Can you work these out from the model? Positions are in its coordinate system, mm. Face numbers are marked on the shaded views. A direction names the side the tool comes from. Round coordinates to 2 decimals unless told otherwise and drop trailing zeros. Loops run counter-clockwise (first coordinate to the right, second up) from the corner with the lowest first, then second, coordinate; pieces in that order, holes last. Notation, with made-up numbers: (33.5, 2.25) -> (89.5, 2.25) arc R21 cw to (89.5, 8.25) -> close; hole circle Ø6 at (14, 46.25). An arc over 180 degrees is marked (long way). Use a Markdown table: item, result.
from build123d import *

# Parameters (mm, degrees)
SKETCH_3_W           = 180
SKETCH_3_H           = 43
EXTRUDE_1_DEPTH      = 12
CUT_EXTRUDE_1_DEPTH  = 52
CUT_EXTRUDE_2_DEPTH  = 5
CUT_EXTRUDE_3_DEPTH  = 5
SKETCH_8_W           = 55
SKETCH_8_H           = 37
CUT_EXTRUDE_4_DEPTH  = 10.5
CUT_EXTRUDE_5_DEPTH  = 3
SKETCH_10_W          = 62.128790526
SKETCH_10_H          = 8.683746703
CUT_EXTRUDE_6_DEPTH  = 8
CUT_EXTRUDE_8_DEPTH  = 9
FILLET_2_R           = 2
FILLET_3_R           = 3
SKETCH_12_W          = 20
SKETCH_12_H          = 16
EXTRUDE_2_DEPTH      = 2
SKETCH_13_W          = 16
SKETCH_13_H          = 5
CUT_EXTRUDE_9_DEPTH  = 1
SKETCH_14_W          = 10
SKETCH_14_H          = 4.5
CUT_EXTRUDE_10_DEPTH = 11
EXTRUDE_3_DEPTH      = 2
EXTRUDE_3_DEPTH_BACK = 3
SKETCH_15_W          = 4.878003414
SKETCH_15_H          = 8.248491994


with BuildPart() as part:
    # 草图3 → 凸台-拉伸1 (new body)
    with BuildSketch(Plane(origin=(0, 0, 0), x_dir=(1, 0, 0), z_dir=(0, 1, 0))):
        with Locations((50.068597249, 7.753123643)):
            Rectangle(SKETCH_3_W, SKETCH_3_H)
    extrude(amount=EXTRUDE_1_DEPTH)

    # 草图4 → 切除-拉伸1 (cut)
    with BuildSketch(Plane(origin=(0, 0, 0), x_dir=(1, 0, 0), z_dir=(0, 1, 0))):
        Polygon((-22.469613434, -5.858946979), (26.002261286, -5.858946979), (29.068597249, -13.746876357), (-25.931402751, -13.746876357), align=None)
    extrude(amount=CUT_EXTRUDE_1_DEPTH, mode=Mode.SUBTRACT)

    # 草图5 → 切除-拉伸2 (cut)
    with BuildSketch(Plane(origin=(0, 12, 0), x_dir=(1, 0, 0), z_dir=(0, 1, 0))):
        Polygon((140.068597249, 7.753123643), (140.068597249, 22.753123643), (125.276479966, 22.753123643), (125.276479966, -7.246876357), (140.068597249, -7.246876357), align=None)
    extrude(amount=-CUT_EXTRUDE_2_DEPTH, mode=Mode.SUBTRACT)

    # 草图7 → 切除-拉伸3 (cut)
    with BuildSketch(Plane(origin=(0, 12, 0), x_dir=(1, 0, 0), z_dir=(0, 1, 0))):
        Polygon((125.276479966, 7.753123643), (125.276479966, 25.753123643), (100.500825538, 25.753123643), (100.500825538, -10.246876357), (125.276479966, -10.246876357), align=None)
    extrude(amount=-CUT_EXTRUDE_3_DEPTH, mode=Mode.SUBTRACT)

    # 草图8 → 切除-拉伸4 (cut)
    with BuildSketch(Plane(origin=(0, 12, 0), x_dir=(1, 0, 0), z_dir=(0, 1, 0))):
        with Locations((63.776287419, 7.753123643)):
            Rectangle(SKETCH_8_W, SKETCH_8_H)
    extrude(amount=-CUT_EXTRUDE_4_DEPTH, mode=Mode.SUBTRACT)

    # 草图9 → 切除-拉伸5 (cut)
    with BuildSketch(Plane(origin=(0, 12, 0), x_dir=(1, 0, 0), z_dir=(0, 1, 0))):
        Polygon((91.276287419, 26.253123643), (96.635770173, 26.253123643), (96.635770173, 22.130591531), (96.635770173, 13.862098754), (97.813575381, 11.877191358), (100.500825538, 11.877191358), (100.500825538, 3.393971617), (96.236747254, 3.393971617), (92.132656028, 10.310430274), (92.132656028, 21.255120764), (91.276287419, 21.255120764), align=None)
    extrude(amount=-CUT_EXTRUDE_5_DEPTH, mode=Mode.SUBTRACT)

    # 草图10 → 切除-拉伸6 (cut)
    with BuildSketch(Plane(origin=(0, 12, 0), x_dir=(1, 0, 0), z_dir=(0, 1, 0))):
        with Locations((1.934159822, -6.405003006)):
            Rectangle(SKETCH_10_W, SKETCH_10_H)
    extrude(amount=-CUT_EXTRUDE_6_DEPTH, mode=Mode.SUBTRACT)

    # 草图11 → 切除-拉伸8 (cut)
    with BuildSketch(Plane(origin=(0, 12, 0), x_dir=(1, 0, 0), z_dir=(0, 1, 0))):
        Polygon((32.998555085, -10.746876357), (-36.5396752, -10.746876357), (-36.5396752, 26.253123643), (36.276287419, 26.253123643), (36.276287419, -2.167243749), (32.998555085, -2.063129654), align=None)
    extrude(amount=-CUT_EXTRUDE_8_DEPTH, mode=Mode.SUBTRACT)

    # 圆角2
    fillet_2_edges = [part.edges().sort_by_distance(p)[0] for p in [
        (84.568597249, 0, 13.746876357),
        (-24.200508092, 0, 9.802911668),
        (27.535429268, 0, 9.802911668),
        (50.068597249, 0, -29.253123643),
        (140.068597249, 0, -7.753123643),
        (-32.931402751, 0, 13.746876357),
        (-39.931402751, 0, -7.753123643),
    ]]
    fillet(fillet_2_edges, radius=FILLET_2_R)

    # 圆角3
    # the kernel refuses this fillet: 3 mm, written as the material it takes off along each edge
    with BuildSketch(Plane(origin=(-36.931402751, 0, 10.746876357), x_dir=(0, 0, 1), z_dir=(1, 0, 0))) as fillet_3_piece_1:
        with BuildLine():
            CenterArc((1, -2), 2, 0, 90)
            Line((3, -2), (3, 0))
            Line((3, 0), (1, 0))
        make_face()
    revolve(axis=Axis((-36.931402751, 0, 10.746876357), (0, -1, 0)), revolution_arc=90, mode=Mode.SUBTRACT)
    with BuildSketch(Plane(origin=(-36.931402751, 0, -26.253123643), x_dir=(-1, 0, 0), z_dir=(0, 0, 1))) as fillet_3_piece_2:
        with BuildLine():
            CenterArc((1, -2), 2, 0, 90)
            Line((3, -2), (3, 0))
            Line((3, 0), (1, 0))
        make_face()
    revolve(axis=Axis((-36.931402751, 0, -26.253123643), (0, -1, 0)), revolution_arc=90, mode=Mode.SUBTRACT)
    with BuildSketch(Plane(origin=(137.068597249, 0, 10.746876357), x_dir=(1, 0, 0), z_dir=(0, 0, -1))) as fillet_3_piece_3:
        with BuildLine():
            CenterArc((1, -2), 2, 0, 90)
            Line((3, -2), (3, 0))
            Line((3, 0), (1, 0))
        make_face()
    revolve(axis=Axis((137.068597249, 0, 10.746876357), (0, -1, 0)), revolution_arc=90, mode=Mode.SUBTRACT)
    with BuildSketch(Plane(origin=(137.068597249, 0, -26.253123643), x_dir=(0, 0, -1), z_dir=(-1, 0, 0))) as fillet_3_piece_4:
        with BuildLine():
            CenterArc((1, -2), 2, 0, 90)
            Line((3, -2), (3, 0))
            Line((3, 0), (1, 0))
        make_face()
    revolve(axis=Axis((137.068597249, 0, -26.253123643), (0, -1, 0)), revolution_arc=90, mode=Mode.SUBTRACT)
    with BuildSketch(Plane(origin=(-39.931402751, 0, -29.253123643), x_dir=(1, 0, 0), z_dir=(0, 1, 0))) as fillet_3_piece_5:
        with BuildLine():
            CenterArc((FILLET_3_R, -FILLET_3_R), FILLET_3_R, 90, 90)
            Line((0, -FILLET_3_R), (0, 0))
            Line((0, 0), (FILLET_3_R, 0))
        make_face()
    extrude(amount=19.5, mode=Mode.SUBTRACT)
    with BuildSketch(Plane(origin=(140.068597249, 0, -29.253123643), x_dir=(-1, 0, 0), z_dir=(0, 1, 0)), Plane(origin=(140.068597249, 0, 13.746876357), x_dir=(0, 0, -1), z_dir=(0, 1, 0)), Plane(origin=(-39.931402751, 0, 13.746876357), x_dir=(1, 0, 0), z_dir=(0, 1, 0))) as fillet_3_piece_6:
        with BuildLine():
            CenterArc((FILLET_3_R, FILLET_3_R), FILLET_3_R, 180, 90)
            Line((0, FILLET_3_R), (0, 0))
            Line((0, 0), (FILLET_3_R, 0))
        make_face()
    extrude(amount=19.5, mode=Mode.SUBTRACT)

    # 草图12 → 凸台-拉伸2 (add)
    with BuildSketch(Plane(origin=(0, 3, 0), x_dir=(1, 0, 0), z_dir=(0, 1, 0))):
        with Locations((-26.5396752, 11.082072108)):
            Rectangle(SKETCH_12_W, SKETCH_12_H)
    extrude(amount=EXTRUDE_2_DEPTH)

    # 草图13 → 切除-拉伸9 (cut)
    with BuildSketch(Plane(origin=(-36.5396752, 0, 0), x_dir=(0, 0, -1), z_dir=(1, 0, 0))):
        with Locations((11.082072108, 7.5)):
            Rectangle(SKETCH_13_W, SKETCH_13_H)
    extrude(amount=-CUT_EXTRUDE_9_DEPTH, mode=Mode.SUBTRACT)

    # 草图14 → 切除-拉伸10 (cut)
    with BuildSketch(Plane(origin=(-37.5396752, 0, 0), x_dir=(0, 0, -1), z_dir=(1, 0, 0))):
        with Locations((11.082072108, 7.25)):
            Rectangle(SKETCH_14_W, SKETCH_14_H)
    extrude(amount=-CUT_EXTRUDE_10_DEPTH, mode=Mode.SUBTRACT)

    # 草图15 → 凸台-拉伸3 (add, two sides: drawn at the far end of the back side and taken through both)
    with BuildSketch(Plane(origin=(0, 5, 0), x_dir=(1, 0, 0), z_dir=(0, 1, 0)).offset(-EXTRUDE_3_DEPTH_BACK)):
        with Locations((-8.100673493, 11.957826111)):
            Rectangle(SKETCH_15_W, SKETCH_15_H)
    extrude(amount=EXTRUDE_3_DEPTH + EXTRUDE_3_DEPTH_BACK)


solid = part.part
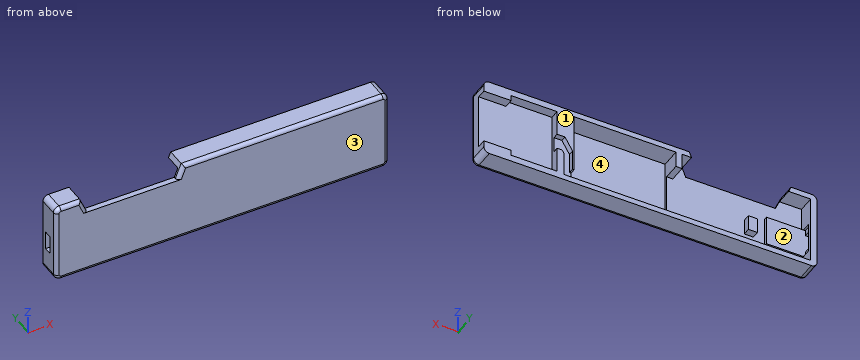
1. Which directions (+Z, -Z, +X, -X, +Y, -Y) give clear straight access to the entire face, cutting with the end or side of a thin tool? Please do the marked faces 3 and 4.
Answer sheet:
| item | result |
|---|---|
| face 3 | +Z, -Z, +X, -X, -Y |
| face 4 | +Y |
2. I want a section at B-B (x = 80). Please give me the cut outline in (y, z).
Answer sheet:
| item | result |
|---|---|
| outline | (0, -27.25) arc R2 ccw to (2, -29.25) -> (12, -29.25) -> (12, -26.25) -> (1.5, -26.25) -> (1.5, 10.75) -> (12, 10.75) -> (12, 13.75) -> (2, 13.75) arc R2 ccw to (0, 11.75) -> close |
3. I want a section at A-A (x = 5). Please give me the cut outline in (y, z), plus the area to 3 significant figures.
Answer sheet:
| item | result |
|---|---|
| outline | (0, -27.25) arc R2 ccw to (2, -29.25) -> (12, -29.25) -> (12, -26.25) -> (3, -26.25) -> (3, 5.86) -> (0, 5.86) -> close |
| area | 131 mm² |
4. Will these pins go through, and if not, where does the flat tip stop? pin 1 Ø2.5 at (x, z) = (-7.5, -13) entering from +Y; pin 2 Ø13 at (x, z) = (-27, -10) entering from +Y; pin 3 Ø1.9 at (x, y) = (-39, 7.5) entering from +Z.
Answer sheet:
| item | result |
|---|---|
| pin 1 | stops at y = 7 |
| pin 2 | stops at y = 5 |
| pin 3 | stops at z = 13.53 |
5. I want a section at C-C (x = 119). Please give me the cut outline in (y, z).
Answer sheet:
| item | result |
|---|---|
| outline | (0, -27.25) arc R2 ccw to (2, -29.25) -> (12, -29.25) -> (12, -25.75) -> (7, -25.75) -> (7, 10.25) -> (12, 10.25) -> (12, 13.75) -> (2, 13.75) arc R2 ccw to (0, 11.75) -> close |
6. I need wall thicknesses on line 1 (X direction, y = 9.5, z = -18); line 2 (X direction, y = 3.75, z = -5); line 3 (X direction, y = 11.25, z = 1). Which ranges of each line are inside material? Lowest first, please.
Answer sheet:
| item | result |
|---|---|
| line 1 | x = -39.93 to -37.54, 91.28 to 92.13, 96.64 to 100.5 |
| line 2 | x = -39.93 to -16.54, 91.28 to 140.07 |
| line 3 | x = -39.93 to -36.54, 91.28 to 100.5 |
7. If we mould it in two halves opening along Z, with no side actions, what happens to the marked faces 1 and 2? For each: +Z half, -Z half, draft (parallel to the pull), parting line (faces both ways), or undercut.
Answer sheet:
| item | result |
|---|---|
| face 1 | draft |
| face 2 | undercut |
